```python
from build123d import *

# Parameters (mm, degrees)
SALIENTE_EXTRUIR1_DEPTH      = 35
SALIENTE_EXTRUIR1_DEPTH_BACK = 35
CORTAR_EXTRUIR1_DEPTH        = 3
CROQUIS4_R                   = 8
CORTAR_EXTRUIR2_DEPTH        = 3
CROQUIS5_R                   = 2.5
CORTAR_EXTRUIR3_DEPTH        = 10
CROQUIS6_W                   = 6
CROQUIS6_H                   = 10
CORTAR_EXTRUIR5_DEPTH        = 10
CROQUIS7_W                   = 2
CROQUIS7_H                   = 2
CORTAR_EXTRUIR6_DEPTH        = 5
CROQUIS8_R                   = 1
CORTAR_EXTRUIR7_DEPTH        = 2
CROQUIS9_W                   = 6
CROQUIS9_H                   = 10
CORTAR_EXTRUIR8_DEPTH        = 12
CORTAR_EXTRUIR9_DEPTH        = 5
CORTAR_EXTRUIR9_DEPTH_BACK   = 5
CROQUIS10_R                  = 1
CORTAR_EXTRUIR10_DEPTH       = 5
CORTAR_EXTRUIR10_DEPTH_BACK  = 5
CORTAR_EXTRUIR11_DEPTH       = 3
CORTAR_EXTRUIR11_DEPTH_BACK  = 3
CROQUIS14_W                  = 2
CROQUIS14_H                  = 10
SALIENTE_EXTRUIR2_DEPTH      = 5
CROQUIS15_R                  = 2.5
CORTAR_EXTRUIR12_DEPTH       = 15


with BuildPart() as part:
    # Croquis1 → Saliente-Extruir1 (new, two sides: drawn at the far end of the back side and taken through both)
    with BuildSketch(Plane.XY.offset(-SALIENTE_EXTRUIR1_DEPTH_BACK)):
        with BuildLine():
            Line((-15, 0), (15, 0))
            ThreePointArc((15, 0), (0, -15), (-15, 0))
        make_face()
    extrude(amount=SALIENTE_EXTRUIR1_DEPTH + SALIENTE_EXTRUIR1_DEPTH_BACK)

    # Croquis3 → Cortar-Extruir1 (cut)
    with BuildSketch(Plane(origin=(0, 0, 0), x_dir=(1, 0, 0), z_dir=(0, 1, 0))):
        with BuildLine():
            Line((-8, 25), (-12.284525276, 15.598253186))
            ThreePointArc((-12.284525276, 15.598253186), (0, -3.5), (12.284525276, 15.598253186))
            Line((12.284525276, 15.598253186), (8, 25))
            ThreePointArc((8, 25), (13, 30), (8, 35))
            Line((8, 35), (-8, 35))
            ThreePointArc((-8, 35), (-13, 30), (-8, 25))
        make_face()
    extrude(amount=-CORTAR_EXTRUIR1_DEPTH, mode=Mode.SUBTRACT)

    # Croquis4 → Cortar-Extruir2 (cut)
    with BuildSketch(Plane(origin=(0, -3, 0), x_dir=(1, 0, 0), z_dir=(0, 1, 0))):
        with Locations(Location((0, 10, 0), (0, 0, 270))):
            Circle(CROQUIS4_R)
    extrude(amount=-CORTAR_EXTRUIR2_DEPTH, mode=Mode.SUBTRACT)

    # Croquis5 → Cortar-Extruir3 (cut)
    with BuildSketch(Plane(origin=(0, -6, 0), x_dir=(1, 0, 0), z_dir=(0, 1, 0))):
        with Locations(Location((0, 10, 0), (0, 0, 270))):
            Circle(CROQUIS5_R)
    extrude(amount=-CORTAR_EXTRUIR3_DEPTH, mode=Mode.SUBTRACT)

    # Croquis6 → Cortar-Extruir5 (cut)
    with BuildSketch(Plane(origin=(0, -3, 0), x_dir=(1, 0, 0), z_dir=(0, 1, 0))):
        with Locations((0, 30)):
            Rectangle(CROQUIS6_W, CROQUIS6_H)
    extrude(amount=-CORTAR_EXTRUIR5_DEPTH, mode=Mode.SUBTRACT)

    # Croquis7 → Cortar-Extruir6 (cut)
    with BuildSketch(Plane(origin=(0, -3, 0), x_dir=(1, 0, 0), z_dir=(0, 1, 0))):
        with Locations((-4, 30)):
            Rectangle(CROQUIS7_W, CROQUIS7_H)
        with Locations((4, 30)):
            Rectangle(CROQUIS7_W, CROQUIS7_H)
    extrude(amount=-CORTAR_EXTRUIR6_DEPTH, mode=Mode.SUBTRACT)

    # Croquis8 → Cortar-Extruir7 (cut)
    with BuildSketch(Plane(origin=(0, -3, 0), x_dir=(1, 0, 0), z_dir=(0, 1, 0))):
        with Locations(Location((-8, 30, 0), (0, 0, 270))):
            Circle(CROQUIS8_R)
        with Locations(Location((8, 30, 0), (0, 0, 270))):
            Circle(CROQUIS8_R)
    extrude(amount=-CORTAR_EXTRUIR7_DEPTH, mode=Mode.SUBTRACT)

    # Croquis9 → Cortar-Extruir8 (cut)
    with BuildSketch(Plane(origin=(0, -3, 0), x_dir=(1, 0, 0), z_dir=(0, 1, 0))):
        Rectangle(CROQUIS9_W, CROQUIS9_H)
    extrude(amount=-CORTAR_EXTRUIR8_DEPTH, mode=Mode.SUBTRACT)

    # Croquis10 → Cortar-Extruir9 (cut, two sides: drawn at the far end of the back side and taken through both)
    with BuildSketch(Plane(origin=(0, 0, 0), x_dir=(0, 0, -1), z_dir=(1, 0, 0)).offset(-CORTAR_EXTRUIR9_DEPTH_BACK)):
        with Locations((30, -8)):
            Circle(CROQUIS10_R)
    extrude(amount=CORTAR_EXTRUIR9_DEPTH + CORTAR_EXTRUIR9_DEPTH_BACK, mode=Mode.SUBTRACT)

    # Croquis11 → Cortar-Extruir10 (cut, two sides: drawn at the far end of the back side and taken through both)
    with BuildSketch(Plane(origin=(0, 0, 0), x_dir=(0, 0, -1), z_dir=(1, 0, 0)).offset(-CORTAR_EXTRUIR10_DEPTH_BACK)):
        with BuildLine():
            Line((-6, -15), (6, -15))
            Line((6, -15), (6, -14))
            Line((6, -14), (1, -14))
            Line((1, -14), (1, -8))
            ThreePointArc((1, -8), (0, -7), (-1, -8))
            Line((-1, -8), (-1, -14))
            Line((-1, -14), (-6, -14))
            Line((-6, -14), (-6, -15))
        make_face()
    extrude(amount=CORTAR_EXTRUIR10_DEPTH + CORTAR_EXTRUIR10_DEPTH_BACK, mode=Mode.SUBTRACT)

    # Croquis12 → Cortar-Extruir11 (cut, two sides: drawn at the far end of the back side and taken through both)
    with BuildSketch(Plane(origin=(0, 0, 0), x_dir=(0, 0, -1), z_dir=(1, 0, 0)).offset(-CORTAR_EXTRUIR11_DEPTH_BACK)):
        with BuildLine():
            Line((-3, -13), (-21.658767316, -9.861464952))
            ThreePointArc((-21.658767316, -9.861464952), (-27.635040051, -6.458030924), (-30, 0))
            Line((-30, 0), (-3, 0))
            Line((-3, 0), (-3, -13))
        make_face()
        Polygon((25, -8), (25, -3), (4, -3), (4, -13), align=None)
    extrude(amount=CORTAR_EXTRUIR11_DEPTH + CORTAR_EXTRUIR11_DEPTH_BACK, mode=Mode.SUBTRACT)

    # Croquis14 → Saliente-Extruir2 (add)
    with BuildSketch(Plane(origin=(0, 0, 0), x_dir=(1, 0, 0), z_dir=(0, 1, 0))):
        with Locations((4, -20)):
            Rectangle(CROQUIS14_W, CROQUIS14_H)
        with Locations((-4, -20)):
            Rectangle(CROQUIS14_W, CROQUIS14_H)
    extrude(amount=SALIENTE_EXTRUIR2_DEPTH)

    # Croquis15 → Cortar-Extruir12 (cut)
    with BuildSketch(Plane(origin=(0, 0, 0), x_dir=(0, 0, -1), z_dir=(1, 0, 0))):
        with Locations((-20, 0)):
            Circle(CROQUIS15_R)
    extrude(amount=CORTAR_EXTRUIR12_DEPTH, mode=Mode.SUBTRACT)


solid = part.part
```
Read the model definition and answer for the solid it produces. Units are mm, in the model's axes. A direction names the side the tool comes from. Coordinates: 2 decimals unless noted, no trailing zeros. Write each loop counter-clockwise with the first axis right and the second up, starting at its lowest first coordinate (ties: lowest second). Pieces come first, ordered by that corner, then holes. Notation, with made-up numbers: (10.5, 5.25) -> (60.5, 5.25) arc R21 ccw to (60.5, 36.25) -> close; hole circle Ø7 at (6, 33.25). An arc over 180 degrees is marked (long way). Return JSON: item names as keys, results as strings.
1. A cutting plane is placed at A-A (z = -26). Determine the outline of the cut face in (x, y).
Found:
{"outline": "(-15, 0) arc R15 ccw to (15, 0) -> (11, 0) -> (11, -3) -> (3, -3) -> (3, -13) -> (-3, -13) -> (-3, -3) -> (-11, -3) -> (-11, 0) -> close"}
2. A cutting plane is placed at C-C (z = 0). Determine the outline of the cut face in (x, y), and give its area (3 significant figures).
Found:
{"outline": "(-15, 0) arc R15 ccw to (-5, -14.14) -> (-5, -7) -> (-3, -7) -> (-3, -3) -> (-9.07, -3) -> (-9.07, 0) -> close; (3, -7) -> (5, -7) -> (5, -14.14) arc R15 ccw to (15, 0) -> (9.07, 0) -> (9.07, -3) -> (3, -3) -> close", "area": "198 mm2"}
3. A cutting plane is placed at B-B (x = 0). Determine the outline of the cut face in (y, z).
Found:
{"outline": "(-15, -35) -> (-13, -35) -> (-13, -25) -> (-8, -25) -> (-10.98, -12.5) -> (-15, -12.5) -> close; (-15, -7.5) -> (-12.17, -7.5) -> (-12.76, -5) -> (-14, -5) -> (-14, -6) -> (-15, -6) -> close; (-15, 6) -> (-14, 6) -> (-14, 5) -> (-12.66, 5) -> (-9.86, 21.66) arc R10 cw to (0, 30) -> (0, 35) -> (-15, 35) -> close"}
4. Determine the mould class of faces 5 (the face through (-5, 2, 20)), 6 (the face through (5.44, -13.98, -0.49)), 7 (the face through (0, -13, -5)), 8 (the face through (-4, 2, 25)) for opening direction X: pulls with the +X half, pulls with the -X half, needs draft (parallel to the pull), parting line crosses it, or undercut.
Found:
{"face 5": "pulls with the -X half", "face 6": "parting line crosses it", "face 7": "undercut", "face 8": "needs draft"}
5. A tool of negligible diameter and unlimited length cuts with its end or side. For faces 1 (the face through (0.1, -13.4, -12.5)), 2 (the face through (-5, -11, 0)), 3 (the face through (8, -3, -16)), 4 (the face through (7.58, -2.44, 20.54)), from which of +Z, -Z, +X, -X, +Y, -Y can it reach the whole face along a straight path? Write none if from no direction.
Found:
{"face 1": "+Y, -Y", "face 2": "-Y", "face 3": "+Y", "face 4": "+X"}
6. Each of these flat-tipped pins is pushed along its axis until it touches: P1, Ø3, axis at y = -5, z = -9.5, coming from the +X side; P2, Ø12, axis at x = -11, z = -7.5, coming from the -Y side; P3, Ø1, axis at x = 10, z = -9.5, coming from the +Y side. Where does it stop, or does it pass through?
Found:
{"P1": "x = 14.59", "P2": "y = -14.14", "P3": "y = -3"}
7. A cutting plane is placed at D-D (x = 11.5). Determine the outline of the cut face in (y, z).
Found:
{"outline": "(-9.63, -35) -> (0, -35) -> (0, -33.57) -> (-3, -33.57) -> (-3, -26.43) -> (0, -26.43) -> (0, -17.32) -> (-3, -17.32) -> (-3, -2.93) -> (0, -2.93) -> (0, 17.5) arc R2.5 cw to (0, 22.5) -> (0, 35) -> (-9.63, 35) -> close"}
8. Find the intervals of material crossed by line 1 along Y through (x, z) = (12, 20); line 2 along X through (y, z) = (-4.1, -30); line 3 along X through (y, z) = (-6, -20), in increasing order. Write a range as from..to.
Found:
{"line 1": "-9..-2.5", "line 2": "-14.43..-9, -7..-5, 5..7, 9..14.43", "line 3": "-13.75..-3, 3..13.75"}
